```python
from build123d import *

# Parameters (mm, degrees)
BOSS_EXTRUDE1_DEPTH = 25.4
FILLET1_R           = 0.8
SKETCH2_R           = 2.0193
CUT_EXTRUDE1_DEPTH  = 50.8


with BuildPart() as part:
    # Sketch1 → Boss-Extrude1 (new body)
    with BuildSketch(Plane.XY):
        Polygon((0, 0), (0, 38.1), (-22.225, 0), align=None)
    extrude(amount=BOSS_EXTRUDE1_DEPTH)

    # Fillet1
    fillet1_edges = [part.edges().sort_by_distance(p)[0] for p in [
        (-11.1125, 19.05, 25.4),
        (-11.1125, 19.05, 0),
        (0, 19.05, 0),
        (-11.1125, 0, 0),
        (-11.1125, 0, 25.4),
        (-22.225, 0, 12.7),
        (0, 38.1, 12.7),
        (0, 0, 12.7),
        (0, 19.05, 25.4),
    ]]
    fillet(fillet1_edges, radius=FILLET1_R)

    # Sketch2 → Cut-Extrude1 (cut)
    with BuildSketch(Plane(origin=(0, 0, 0), x_dir=(0, 0, -1), z_dir=(1, 0, 0))):
        with Locations((-12.7, 26.885863544)):
            Circle(SKETCH2_R)
        with Locations((-12.7, 7.835863544)):
            Circle(SKETCH2_R)
    extrude(amount=-CUT_EXTRUDE1_DEPTH, mode=Mode.SUBTRACT)


solid = part.part
```
Can you work these out from the model? Positions are in its coordinate system, mm. Give positions to 0.01 mm unless a question says otherwise; leave off trailing zeros. Order: outer loops, then holes, each group sorted by start corner. A loop starts at its lowest first (then second) coordinate and runs counter-clockwise, first axis right, second up. Notation, with made-up numbers: M 65,-11.5 L 86,-11.5 A19 cw 86,14.5 Z; hole C -1.75,58 d10. An arc over 180 degrees is marked long. One line per item, written item: value.
1) We'd pull the mould along Y, two halves only. Please class faces 1 (the face through (-11.45, 18.02, 0.24)), 2 (the face through (-9.298, 6.044, 11.768)), 3 (the face through (-0.23, 18.21, 25.16)): released by +Y, released by -Y, zero draft, split by the parting line, or undercut.
Answer sheet:
face 1: released by +Y
face 2: undercut
face 3: zero draft
2) For P1, Ø4.5, axis at y = 26.89, z = 12.7, coming from the -X side; P2, Ø1.5, axis at y = 22, z = 8.5, coming from the -X side; P3, Ø4, axis at y = 7, z = 19.5, coming from the -X side, each with a flat end and sliding along its axis, tell me the tip position at first contact or that it passes through.
Answer sheet:
P1: stops at x = -7.85
P2: stops at x = -9.83
P3: stops at x = -19.31
3) Please list where these lines run through material, in increasing order: line 1 along Y through (x, z) = (-6.75, 12.7); line 2 along Y through (x, z) = (-4, 12.7); line 3 along Y through (x, z) = (-5.25, 12.7).
Answer sheet:
line 1: y = 0 to 5.82, 9.86 to 24.87
line 2: y = 0 to 5.82, 9.86 to 24.87, 28.91 to 31.24
line 3: y = 0 to 5.82, 9.86 to 24.87, 28.91 to 29.1
4) I want a section at C-C, the plane x = -3.5. Count the separate pieces of the cut face and the enclosed holes in it, plus the area to 3 significant figures.
Answer sheet:
separate pieces: 1
enclosed holes: 2
area: 789 mm^2
5) I want a section at B-B, the plane z = 12.7. List the corners of the cut face in (x, y) for me.
Answer sheet:
outline: M -21.52,1.2 A0.8 ccw -20.83,0 L -0.8,0 A0.8 ccw 0,0.8 L 0,5.82 L -18.83,5.82 Z; M -16.48,9.86 L 0,9.86 L 0,24.87 L -7.72,24.87 Z; M -5.36,28.91 L 0,28.91 L 0,35.14 A0.8 ccw -1.49,35.54 Z
6) I want a section at A-A, the plane z = 4. List the corners of the cut face in (x, y) for me.
Answer sheet:
outline: M -21.52,1.2 A0.8 ccw -20.83,0 L -0.8,0 A0.8 ccw 0,0.8 L 0,35.14 A0.8 ccw -1.49,35.54 Z
